For this review, use the dimensioned drawing (mm, ordinates from the lowest corner) and the shaded views. A direction names the side the tool comes from. Coordinates: 2 decimals unless noted, no trailing zeros. Write each loop counter-clockwise with the first axis right and the second up, starting at its lowest first coordinate (ties: lowest second). Pieces come first, ordered by that corner, then holes. Notation, with made-up numbers: (35, -32.75) -> (72, -32.75) arc R35 ccw to (72, 2.25) -> close; hole circle Ø3 at (51.25, 63). An arc over 180 degrees is marked (long way). Return JSON: item names as keys, results as strings. Group by question number.
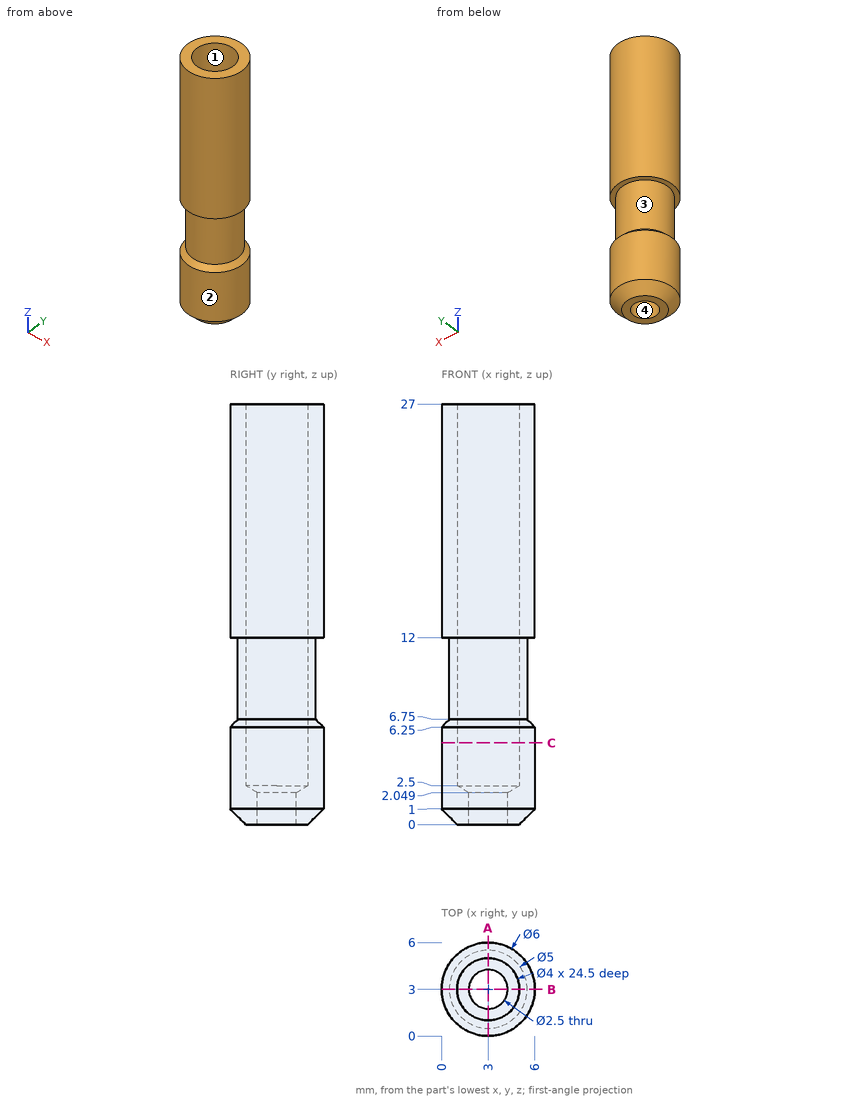
Q1. We need section A-A on x = 3. Write out the cut boundary in (y, z).
Q2. For P1, Ø1, axis at x = 4, y = 3.5, coming from the -Z side; P2, Ø3, axis at x = 3, y = 3, coming from the +Z side; P3, Ø2, axis at x = 1, y = 0.5, coming from the -Z side, all flat-tipped, find the tip position at first contact; note any pin that passes through.
Q3. The part is to be moulded in two halves that separate along X. For the marked faces 3 and 4, say which applies: +X half, -X half, draft (parallel to the pull), parting line (faces both ways), or undercut.
Q4. For the marked faces 1 and 2, list the 3-axis set-ups (+Z, -Z, +X, -X, +Y, -Y) from which the entire face can be reached by the end or side of a thin tool; tool diameter is ignored.
Q5. Wall thickness on L1, parallel to X at y = 3, z = 17.75; L2, parallel to Y at x = 3, z = 8: over which ranges is each line inside the solid? List them lowest first.
Q6. We need section C-C on z = 5.25. Write out the cut boundary in (x, y).
Findings below:
{
 "1": {"outline": "(0, 1) -> (1, 0) -> (1.75, 0) -> (1.75, 2.05) -> (1, 2.5) -> (1, 27) -> (0, 27) -> (0, 12) -> (0.5, 12) -> (0.5, 6.75) -> (0, 6.25) -> close; (4.25, 0) -> (5, 0) -> (6, 1) -> (6, 6.25) -> (5.5, 6.75) -> (5.5, 12) -> (6, 12) -> (6, 27) -> (5, 27) -> (5, 2.5) -> (4.25, 2.05) -> close"},
 "2": {"P1": "stops at z = 0", "P2": "stops at z = 2.2", "P3": "stops at z = 0.2"},
 "3": {"face 3": "parting line", "face 4": "undercut"},
 "4": {"face 1": "+Z", "face 2": "+Z, -Z"},
 "5": {"L1": "x = 0 to 1, 5 to 6", "L2": "y = 0.5 to 1, 5 to 5.5"},
 "6": {"outline": "circle Ø6 at (3, 3); hole circle Ø4 at (3, 3)"}
}
